Can you work these out from the model? Positions are in its coordinate system, mm. Face numbers are marked on the shaded views. A direction names the side the tool comes from. Round coordinates to 2 decimals unless told otherwise and drop trailing zeros. Write each loop counter-clockwise with the first axis right and the second up, starting at its lowest first coordinate (ties: lowest second). Pieces come first, ordered by that corner, then holes. Notation, with made-up numbers: (10.5, 29.25) -> (18.5, 29.25) arc R35 cw to (18.5, 68.25) -> close; hole circle Ø2 at (-40, 23). An arc over 180 degrees is marked (long way). Write item = value, one per line. Start each with the question number.
1) For the marked faces 1, 2 and 3, which set-ups out of +Z, -Z, +X, -X, +Y, -Y let a thin tool reach every point of the face, with its end or its side?
2) Imagine slicing it at A-A, the plane y = 0. Please give me the cut outline in (x, z) (3 decimals), then the cut area to 3 significant figures.
3) Imagine slicing it at B-B, the plane x = -4.5. Please give me the cut outline in (y, z) (3 decimals).
4) If I drill on line 1 (Y direction, x = -4.6, z = 0); line 2 (X direction, y = 4.25, z = 0) (3 decimals); line 3 (Y direction, x = 9, z = -5) (3 decimals), over which ranges is the centre line in solid material (lowest first)?
5) Imagine slicing it at D-D, the plane z = -3.75. Please give me the cut outline in (x, y) (3 decimals).
6) Imagine slicing it at C-C, the plane z = 0. Please give me the cut outline in (x, y) (3 decimals), then the cut area to 3 significant figures.
7) I'm going to push flat-ended pins straight in: pin 1 (3 mm diameter, centred on y = 0.5, z = 0, fed in from +X); pin 2 (3 mm diameter, centred on y = 0.5, z = -0.5, fed in from -X); pin 3 (3 mm diameter, centred on x = -6, z = -0.5, fed in from -Y). Where does each tip first touch, or does it pass through?
8) Thinking about a two-plate mould opening in Y: for the marked faces 4, 5 and 6, which applies, +Y half, -Y half, draft (parallel to the pull), parting line (faces both ways), or undercut?
from build123d import *

# Parameters (mm, degrees)
F0_R     = 1.778
F1_DEPTH = 12.7
F2_R     = 3.175
F3_DEPTH = 12.7
F4_W     = 12.7
F4_H     = 6.35
F5_DEPTH = 12.7
F6_R     = 2.921
F7_DEPTH = 4.064
F8_R     = 3.175
F9_DEPTH = 6.35


with BuildPart() as f1:
    # F0 (on Right) → F1 (new body, symmetric)
    with BuildSketch(Plane.YZ):
        Polygon((-6.35, 3.175), (-6.35, -3.175), (-9.525, -3.175), (-9.525, -6.35), (9.525, -6.35), (9.525, -3.175), (6.35, -3.175), (6.35, 3.175), (9.525, 3.175), (9.525, 6.35), (-9.525, 6.35), (-9.525, 3.175), align=None)
        Circle(F0_R, mode=Mode.SUBTRACT)
    extrude(amount=F1_DEPTH, both=True)

    # F2 (on Front) → F3 (cut, symmetric)
    with BuildSketch(Plane.XZ):
        with Locations((6.35, 0)):
            Circle(F2_R)
    extrude(amount=F3_DEPTH, both=True, mode=Mode.SUBTRACT)

    # F4 (on Top) → F5 (cut, symmetric)
    with BuildSketch(Plane.XY):
        with Locations((6.35, 0)):
            Rectangle(F4_W, F4_H)
    extrude(amount=F5_DEPTH, both=True, mode=Mode.SUBTRACT)

    # F6 (on face) → F7 (cut)
    with BuildSketch(Plane.YZ):
        Circle(F6_R)
    extrude(amount=-F7_DEPTH, mode=Mode.SUBTRACT)

    # F8 (on face) → F9 (cut)
    with BuildSketch(Plane(origin=(-12.7, 0, 0), x_dir=(0, -1, 0), z_dir=(-1, 0, 0))):
        Circle(F8_R)
    extrude(amount=-F9_DEPTH, mode=Mode.SUBTRACT)


solid = f1.part
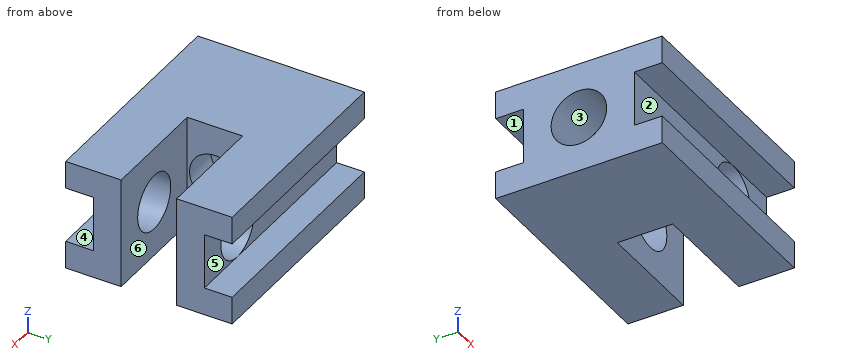
Reported:
q1.face_1 = +X, -X, +Y
q1.face_2 = +X, -X, -Y
q1.face_3 = -X
q2.outline = (-12.7, -6.35) -> (0, -6.35) -> (0, -2.921) -> (-4.064, -2.921) -> (-4.064, -1.778) -> (-6.35, -1.778) -> (-6.35, -3.175) -> (-12.7, -3.175) -> close; (-12.7, 3.175) -> (-6.35, 3.175) -> (-6.35, 1.778) -> (-4.064, 1.778) -> (-4.064, 2.921) -> (0, 2.921) -> (0, 6.35) -> (-12.7, 6.35) -> close
q2.area = 89.1 mm²
q3.outline = (-9.525, -6.35) -> (9.525, -6.35) -> (9.525, -3.175) -> (6.35, -3.175) -> (6.35, 3.175) -> (9.525, 3.175) -> (9.525, 6.35) -> (-9.525, 6.35) -> (-9.525, 3.175) -> (-6.35, 3.175) -> (-6.35, -3.175) -> (-9.525, -3.175) -> close; hole circle Ø3.556 at (0, 0)
q4.line_1 = -6.35 to -1.78, 1.78 to 6.35
q4.line_2 = -12.7 to 3.175, 9.525 to 12.7
q4.line_3 = -9.525 to -3.175, 3.175 to 9.525
q5.outline = (-12.7, -9.525) -> (12.7, -9.525) -> (12.7, -3.175) -> (0, -3.175) -> (0, 3.175) -> (12.7, 3.175) -> (12.7, 9.525) -> (-12.7, 9.525) -> close
q6.outline = (-12.7, -6.35) -> (3.175, -6.35) -> (3.175, -3.175) -> (0, -3.175) -> (0, -2.921) -> (-4.064, -2.921) -> (-4.064, -1.778) -> (-6.35, -1.778) -> (-6.35, -3.175) -> (-12.7, -3.175) -> close; (-12.7, 3.175) -> (-6.35, 3.175) -> (-6.35, 1.778) -> (-4.064, 1.778) -> (-4.064, 2.921) -> (0, 2.921) -> (0, 3.175) -> (3.175, 3.175) -> (3.175, 6.35) -> (-12.7, 6.35) -> close; (9.525, -6.35) -> (12.7, -6.35) -> (12.7, -3.175) -> (9.525, -3.175) -> close; (9.525, 3.175) -> (12.7, 3.175) -> (12.7, 6.35) -> (9.525, 6.35) -> close
q6.area = 129 mm²
q7.pin_1 = -4.06
q7.pin_2 = -6.35
q7.pin_3 = -6.35
q8.face_4 = draft
q8.face_5 = +Y half
q8.face_6 = undercut
